Read the model definition and answer for the solid it produces. Units are mm, in the model's axes. Face numbers are marked on the shaded views. A direction names the side the tool comes from. Coordinates: 2 decimals unless noted, no trailing zeros. Write each loop counter-clockwise with the first axis right and the second up, starting at its lowest first coordinate (ties: lowest second). Pieces come first, ordered by that corner, then holes. Notation, with made-up numbers: (33, 19) - (91, 19) arc R20 ccw to (91, 35) - close; hole circle Ø4 at (46, 5). An arc over 180 degrees is marked (long way). Return JSON: item names as keys, results as strings.
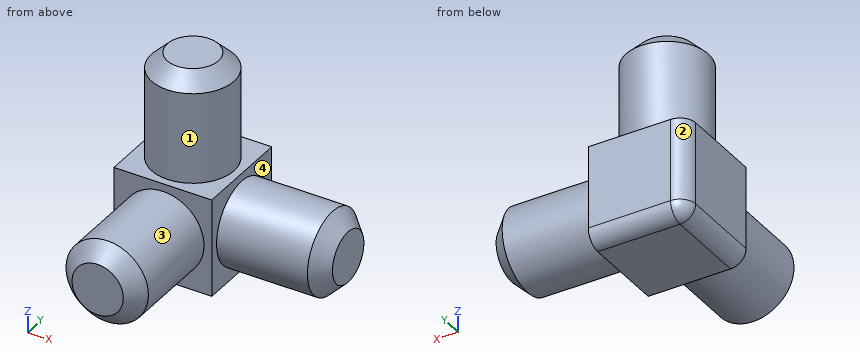
```python
from build123d import *

# Parameters (mm, degrees)
F2_R     = 2.65
F5_DEPTH = 10
F4_R     = 2.65
F6_DEPTH = 10
F3_R     = 2.65
F7_DEPTH = 10
F8_W     = 6.3
F8_H     = 6.3
F9_DEPTH = 3.15
F10_R    = 1
F11_SIZE = 1


with BuildPart() as f5:
    # F2 (on Front) → F5 (new body)
    with BuildSketch(Plane.XZ):
        Circle(F2_R)
    extrude(amount=F5_DEPTH)

    # F4 (on Top) → F6 (join)
    with BuildSketch(Plane.XY):
        Circle(F4_R)
    extrude(amount=F6_DEPTH)

    # F3 (on Right) → F7 (join)
    with BuildSketch(Plane.YZ):
        Circle(F3_R)
    extrude(amount=F7_DEPTH)

    # F8 (on face) → F9 (join, symmetric)
    with BuildSketch(Plane(origin=(0, 0, 0), x_dir=(1, 0, 0), z_dir=(0, 0, -1))):
        Rectangle(F8_W, F8_H)
        with BuildLine():
            Line((-2.65, 0), (0, 0))
            Line((0, 0), (0, -2.65))
            ThreePointArc((0, -2.65), (-1.8738329701, -1.8738329701), (-2.65, 0))
        make_face(mode=Mode.SUBTRACT)
        with BuildLine():
            Line((0, -2.65), (0, 0))
            Line((0, 0), (-2.65, 0))
            ThreePointArc((-2.65, 0), (-1.8738329701, -1.8738329701), (0, -2.65))
        make_face()
    extrude(amount=F9_DEPTH, both=True)

    # F10
    f10_edges = [f5.edges().sort_by_distance(p)[0] for p in [
        (0, 3.15, -3.15),
        (-3.15, 3.15, 0),
        (-3.15, 0, -3.15),
    ]]
    fillet(f10_edges, radius=F10_R)

    # F11
    f11_edges = [f5.edges().sort_by_distance(p)[0] for p in [
        (10, -2.65, 0),
        (-2.65, 0, 10),
        (-2.65, -10, 0),
    ]]
    chamfer(f11_edges, length=F11_SIZE)


solid = f5.part
```
(1) Straight lines are drawn through the part: line 1 (Y direction, x = 6.25, z = 0); line 2 (Z direction, x = 3, y = -1.5); line 3 (Y direction, x = -2, z = 0.5). For each, find the intervals that lie inside material, in ascending order. Write a range as from..to.
Answer:
{"line 1": "-2.65..2.65", "line 2": "-3.15..3.15", "line 3": "-9.59..3.15"}
(2) Which of the six approach directions +Z, -Z, +X, -X, +Y, -Y give full straight-line access (tool end or side, diameter ignored) to the marked faces 1, 2, 3 and 4?
Answer:
{"face 1": "+Z", "face 2": "+Z, -Z, -X, +Y", "face 3": "-Y", "face 4": "+X"}
(3) A cutting plane is placed at C-C (z = 4.75). Determine the outline of the cut face in (x, y).
Answer:
{"outline": "circle Ø5.3 at (0, 0)"}
(4) A cutting plane is placed at A-A (y = 0). Determine the outline of the cut face in (x, z).
Answer:
{"outline": "(-3.15, -2.15) arc R1 ccw to (-2.15, -3.15) - (3.15, -3.15) - (3.15, -2.65) - (9, -2.65) - (10, -1.65) - (10, 1.65) - (9, 2.65) - (3.15, 2.65) - (3.15, 3.15) - (2.65, 3.15) - (2.65, 9) - (1.65, 10) - (-1.65, 10) - (-2.65, 9) - (-2.65, 3.15) - (-3.15, 3.15) - close"}
(5) Flat-ended cylindrical pins translate along their axes: P1, Ø2, axis at x = 2, y = -8.5, coming from the +Z side; P2, Ø4, axis at x = 7, z = 2.5, coming from the -Y side; P3, Ø5, axis at x = 4, z = -2, coming from the -Y side. Find the tip coordinate at first contact, or state that the pin passes through.
Answer:
{"P1": "z = 2.45", "P2": "y = -2.6", "P3": "y = -9.68"}
